Geometry: final body of the model. Coordinates: model frame, mm. Face numbers are marked on the shaded views. A direction names the side the tool comes from. Round coordinates to 2 decimals unless told otherwise and drop trailing zeros. Loops run counter-clockwise (first coordinate to the right, second up) from the corner with the lowest first, then second, coordinate; pieces in that order, holes last. Notation, with made-up numbers: (76.5, -1) -> (119.5, -1) arc R14 cw to (119.5, 5) -> close; hole circle Ø7 at (80, -31). An arc over 180 degrees is marked (long way). Answer in a Markdown table with one row per item.
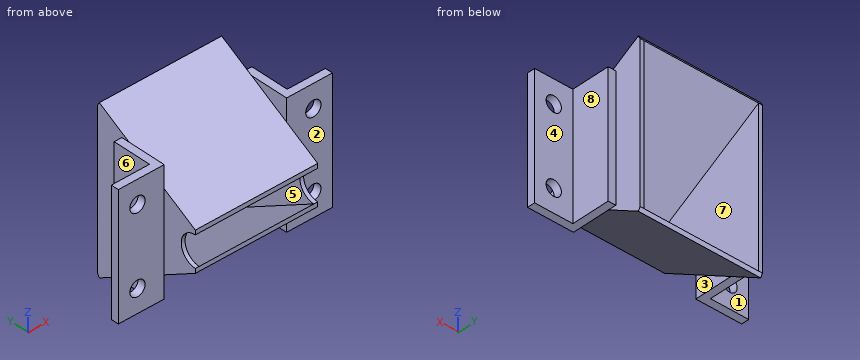
```python
from build123d import *

# Parameters (mm, degrees)
BOSS_EXTRUDE1_DEPTH = 1.5875
SKETCH2_W           = 50.8
SKETCH2_H           = 50.8
BOSS_EXTRUDE2_DEPTH = 1.5875
SKETCH3_W           = 16.36617421
SKETCH3_H           = 0.79375
CUT_EXTRUDE1_DEPTH  = 75.922449176
BOSS_EXTRUDE3_DEPTH = 25.4
SKETCH6_R           = 3.175
CUT_EXTRUDE3_DEPTH  = 81.475374573


with BuildPart() as part:
    # Sketch1 → Boss-Extrude1 (new body)
    with BuildSketch(Plane(origin=(0, 0, 0), x_dir=(0, 0, -1), z_dir=(1, 0, 0))):
        with BuildLine():
            Line((-6.35, 0), (-31.75, 43.994090512))
            Line((-31.75, 43.994090512), (31.75, 43.994090512))
            Line((31.75, 43.994090512), (6.35, 0))
            ThreePointArc((6.35, 0), (0, 6.35), (-6.35, 0))
        make_face()
    boss_extrude1 = extrude(amount=BOSS_EXTRUDE1_DEPTH)

    # Sketch2 → Boss-Extrude2 (add)
    with BuildSketch(Plane(origin=(0, -2.749630657, -4.7625), x_dir=(-1, 0, 0), z_dir=(0, -0.499999999999998, -0.8660254037844397))):
        with Locations((23.8125, 28.575)):
            Rectangle(SKETCH2_W, SKETCH2_H)
    boss_extrude2 = extrude(amount=BOSS_EXTRUDE2_DEPTH)

    # Mirror1: Boss-Extrude2 across plane
    add(boss_extrude2.mirror(Plane.XY))

    # Mirror2: Boss-Extrude1 across plane
    add(boss_extrude1.mirror(Plane(origin=(-23.8125, 0, 0), x_dir=(0, 0, 1), z_dir=(1, 0, 0))))

    # Sketch3 → Cut-Extrude1 (cut, through all)
    with BuildSketch(Plane.ZY.offset(49.2125)):
        with Locations((0, -0.396875)):
            Rectangle(SKETCH3_W, SKETCH3_H)
    extrude(amount=-CUT_EXTRUDE1_DEPTH, mode=Mode.SUBTRACT)

    # Sketch4 → Boss-Extrude3 (add, symmetric)
    with BuildSketch(Plane.XY):
        Polygon((-49.2125, 33.05), (-49.2125, 14), (-68.2625, 14), (-68.2625, 17.175), (-52.3875, 17.175), (-52.3875, 33.05), align=None)
    boss_extrude3 = extrude(amount=BOSS_EXTRUDE3_DEPTH, both=True)

    # Sketch6 → Cut-Extrude3 (cut, through all)
    with BuildSketch(Plane(origin=(0, 17.175, 0), x_dir=(1, 0, 0), z_dir=(0, 1, 0))):
        with Locations(Location((-60.325, 15.875, 0), (0, 0, 270))):
            Circle(SKETCH6_R)
        with Locations(Location((-60.325, -15.875, 0), (0, 0, 270))):
            Circle(SKETCH6_R)
    cut_extrude3 = extrude(amount=-CUT_EXTRUDE3_DEPTH, mode=Mode.SUBTRACT)

    # Mirror3: Boss-Extrude3, Cut-Extrude3 across plane
    add(boss_extrude3.mirror(Plane(origin=(-23.8125, 0, 0), x_dir=(0, 0, 1), z_dir=(1, 0, 0))))
    add(cut_extrude3.mirror(Plane(origin=(-23.8125, 0, 0), x_dir=(0, 0, 1), z_dir=(1, 0, 0))), mode=Mode.SUBTRACT)


solid = part.part
```
Item 1: Draft query along X for the marked faces 6, 7 and 8. Return one class per face: pulls with the +X half, pulls with the -X half, needs draft (parallel to the pull), parting line crosses it, or undercut.
Answer:
| item | result |
|---|---|
| face 6 | pulls with the -X half |
| face 7 | undercut |
| face 8 | pulls with the +X half |
Item 2: Pin query (flat end, axial travel): pin 1 Ø5 at (x, y) = (-8.5, 10) entering from +Z; pin 2 Ø7.5 at (x, z) = (12.7, 15.875) entering from -Y; pin 3 Ø8 at (x, z) = (11.5, -8.5) entering from +Y (3 decimals). Return the tip coordinate at first contact, or that it passes through.
Answer:
| item | result |
|---|---|
| pin 1 | stops at z = 15.4 |
| pin 2 | stops at y = 14 |
| pin 3 | stops at y = 17.175 |
Item 3: Reachability of the marked faces 1, 2, 3, 4 and 5 from +Z, -Z, +X, -X, +Y, -Y: full face, straight path, thin tool, end or side. Return the list, or none.
Answer:
| item | result |
|---|---|
| face 1 | +Z, -Z, -X, +Y |
| face 2 | +Z, -Z, +X, -Y |
| face 3 | -Z, -Y |
| face 4 | +Z, -Z, +X, +Y |
| face 5 | +Y |
Item 4: Cut plane D-D (y = 26). Output: boundary loops of the cut face in (x, z) (1 decimal), then the cut area to 3 significant figures.
Answer:
| item | result |
|---|---|
| outline | (-52.4, -25.4) -> (-49.2, -25.4) -> (-49.2, -23.2) -> (1.6, -23.2) -> (1.6, -25.4) -> (4.8, -25.4) -> (4.8, 25.4) -> (1.6, 25.4) -> (1.6, 23.2) -> (-49.2, 23.2) -> (-49.2, 25.4) -> (-52.4, 25.4) -> close; hole (-47.6, -21.4) -> (0, -21.4) -> (0, 21.4) -> (-47.6, 21.4) -> close |
| area | 644 mm² |
Item 5: Cut plane A-A (x = -8.5). Output: boundary loops of the cut face in (y, z), then the cut area to 3 significant figures.
Answer:
| item | result |
|---|---|
| outline | (0, -8.18) -> (43.2, -33.12) -> (43.99, -31.75) -> (0, -6.35) -> close; (0, 6.35) -> (43.99, 31.75) -> (43.2, 33.12) -> (0, 8.18) -> close |
| area | 160 mm² |
Item 6: Cut plane C-C (x = 12.7). Output: boundary loops of the cut face in (y, z) (3 decimals), then the cut area to 3 significant figures.
Answer:
| item | result |
|---|---|
| outline | (14, -25.4) -> (17.175, -25.4) -> (17.175, -19.05) -> (14, -19.05) -> close; (14, -12.7) -> (17.175, -12.7) -> (17.175, 12.7) -> (14, 12.7) -> close; (14, 19.05) -> (17.175, 19.05) -> (17.175, 25.4) -> (14, 25.4) -> close |
| area | 121 mm² |
Item 7: Line query: probe 1 along X at (y, z) = (25, -11) (1 decimal); probe 2 along X at (y, z) = (34, -23) (1 decimal); probe 3 along Y at (x, z) = (11.5, -5.5) (3 decimals). Output: solid intervals per line, ascending. Write a range as [from, to].
Answer:
| item | result |
|---|---|
| probe 1 | x = [-52.4, -47.6], [0, 4.8] |
| probe 2 | x = [-49.2, -47.6], [0, 1.6] |
| probe 3 | y = [14, 17.175] |
